The listing builds one solid part. Answer for the finished solid, in the listing's coordinates (mm). Face numbers are marked on the shaded views. Give positions to 0.01 mm unless a question says otherwise; leave off trailing zeros. Write each loop counter-clockwise with the first axis right and the second up, starting at its lowest first coordinate (ties: lowest second). Pieces come first, ordered by that corner, then holes. Notation, with made-up numbers: M 31.5,14 L 87.5,14 A11 ccw 87.5,20 Z; hole C 26,82.5 d1. An arc over 180 degrees is marked long. Answer as a JSON object with one key per item and string values.
Autodesk Inventor part; units mm, degrees
ref_plane "Arbeitsebene1" through (0, 0, 12) normal (0, 0, 1) x (1, 0, 0)
ref_plane "YZ Plane" through (0, 0, 0) normal (1, 0, 0) x (0, 1, 0)
ref_plane "XZ Plane" through (0, 0, 0) normal (0, 1, 0) x (-1, 0, 0)
sketch "Skizze1" plane through (0, 0, 0) normal (0, 0, 1) x (1, 0, 0)
  line L0 (-8, -8) -> (8, -8)
  line L1 (8, -8) -> (8, 8)
  line L2 (8, 8) -> (-8, 8)
  line L3 (-8, 8) -> (-8, -8)
extrude "Extrusion1" add sketch "Skizze1" along normal blind 12
sketch "Skizze2" plane through (0, 0, 0) normal (0, 0, 1) x (1, 0, 0)
  circle A0 centre (0, 0) radius 2.2
extrude "Extrusion2" cut sketch "Skizze2" along normal blind 12.2
sketch "Skizze3" plane through (0, 0, 0) normal (0, 0, 1) x (1, 0, 0)
  circle A0 centre (0, 6) radius 1.2
extrude "Extrusion3" cut sketch "Skizze3" along normal blind 12.2
sketch "Skizze4" plane through (0, 0, 0) normal (0, 0, 1) x (1, 0, 0)
  circle A0 centre (0, -6) radius 1.2
extrude "Extrusion4" cut sketch "Skizze4" along normal blind 12.2
ref_plane "Arbeitsebene1" through (0, 0, 12) normal (0, 0, 1) x (1, 0, 0)
sketch "Skizze5" plane through (0, 0, 12) normal (0, 0, 1) x (1, 0, 0)
  circle A0 centre (0, 0) radius 4
extrude "Extrusion5" cut sketch "Skizze5" against normal blind 8
properties part number "Rast_Halter"
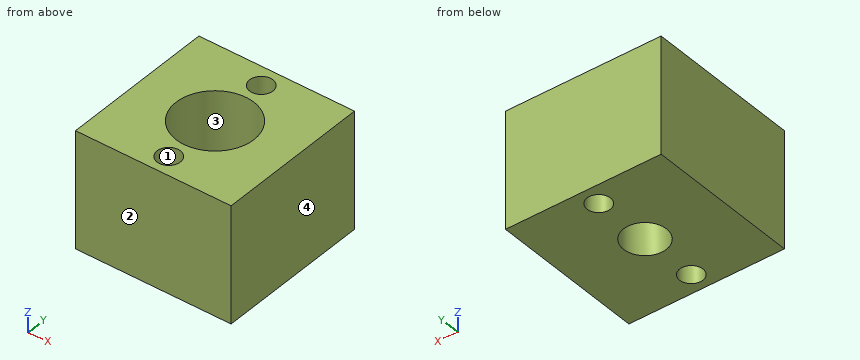
1. The mould has two halves that part along Y. Classify the marked faces 1, 2, 3 and 4: released by +Y, released by -Y, zero draft, split by the parting line, or undercut.
Verdict:
{"face 1": "undercut", "face 2": "released by -Y", "face 3": "undercut", "face 4": "zero draft"}
2. A cutting plane is placed at C-C, the plane y = 6. Give the vertices of the cut face in (x, z), plus the area to 3 significant figures.
Verdict:
{"outline": "M -8,0 L -1.2,0 L -1.2,12 L -8,12 Z; M 1.2,0 L 8,0 L 8,12 L 1.2,12 Z", "area": "163 mm2"}
3. A cutting plane is placed at B-B, the plane x = 0. Give the vertices of the cut face in (y, z), plus the area to 3 significant figures.
Verdict:
{"outline": "M -8,0 L -7.2,0 L -7.2,12 L -8,12 Z; M -4.8,0 L -2.2,0 L -2.2,4 L -4,4 L -4,12 L -4.8,12 Z; M 2.2,0 L 4.8,0 L 4.8,12 L 4,12 L 4,4 L 2.2,4 Z; M 7.2,0 L 8,0 L 8,12 L 7.2,12 Z", "area": "52.8 mm2"}
4. A cutting plane is placed at A-A, the plane z = 10. Give the vertices of the cut face in (x, y), plus the area to 3 significant figures.
Verdict:
{"outline": "M -8,-8 L 8,-8 L 8,8 L -8,8 Z; hole C 0,0 d8; hole C 0,-6 d2.4; hole C 0,6 d2.4", "area": "197 mm2"}
5. A flat-ended cylindrical pin translates along its axis: pin 1 (1.4 mm diameter, centred on x = 0, y = 6, fed in from -Z). Find the tip coordinate at first contact, or state that the pin passes through.
Verdict:
{"pin 1": "passes through"}
6. A cutting plane is placed at D-D, the plane z = 1. Give the vertices of the cut face in (x, y).
Verdict:
{"outline": "M -8,-8 L 8,-8 L 8,8 L -8,8 Z; hole C 0,0 d4.4; hole C 0,-6 d2.4; hole C 0,6 d2.4"}
7. Consider line 1 along Y through (x, z) = (0, 1.5); line 2 along Y through (x, z) = (0, 9.5); line 3 along X through (y, z) = (0, 3). Determine where each line is inside the solid, lowest interval first.
Verdict:
{"line 1": "y = -8 to -7.2, -4.8 to -2.2, 2.2 to 4.8, 7.2 to 8", "line 2": "y = -8 to -7.2, -4.8 to -4, 4 to 4.8, 7.2 to 8", "line 3": "x = -8 to -2.2, 2.2 to 8"}
